Geometry check sheet. Reference: the model listing, model coordinates, mm. A direction names the side the tool comes from. Give positions to 0.01 mm unless a question says otherwise; leave off trailing zeros. Loops run counter-clockwise (first coordinate to the right, second up) from the corner with the lowest first, then second, coordinate; pieces in that order, holes last. Notation, with made-up numbers: (-22.5, -3) -> (29.5, -3) arc R24 ccw to (29.5, 8) -> close; hole circle Ø1 at (73.25, 60). An arc over 180 degrees is marked (long way). Write item = value, one per line. Start each with the question number.
```python
from build123d import *

# Parameters (mm, degrees)
SKETCH1_W           = 253.301246
SKETCH1_H           = 124.905262
BOSS_EXTRUDE1_DEPTH = 13.704316
SKETCH3_R           = 11.68527
BOSS_EXTRUDE6_DEPTH = 133.294628
SKETCH4_R           = 13.935202
BOSS_EXTRUDE7_DEPTH = 24.061166
SKETCH2_R           = 15.942437
BOSS_EXTRUDE8_DEPTH = 14.713204


with BuildPart() as part:
    # Sketch1 → Boss-Extrude1 (new body)
    with BuildSketch(Plane(origin=(0, 0, 0), x_dir=(1, 0, 0), z_dir=(0, 1, 0))):
        Rectangle(SKETCH1_W, SKETCH1_H)
    extrude(amount=BOSS_EXTRUDE1_DEPTH)

    # Sketch3 → Boss-Extrude6 (add)
    with BuildSketch(Plane.XY.offset(66.647314)):
        with Locations((131.1274492, 7.338568)):
            Circle(SKETCH3_R)
    boss_extrude6 = extrude(amount=-BOSS_EXTRUDE6_DEPTH)

    # Sketch4 → Boss-Extrude7 (add)
    with BuildSketch(Plane(origin=(47.4016832, 0, 0), x_dir=(0, 0, -1), z_dir=(1, 0, 0))):
        with BuildLine():
            Line((-44.216574, 0), (44.216574, 0))
            ThreePointArc((44.216574, 0), (0, -44.216574), (-44.216574, 0))
        make_face()
        with Locations(Location((0, -19.057366, 0), (0, 0, 180))):
            Circle(SKETCH4_R, mode=Mode.SUBTRACT)
    boss_extrude7 = extrude(amount=BOSS_EXTRUDE7_DEPTH)

    # Sketch2 → Boss-Extrude8 (add)
    with BuildSketch(Plane(origin=(127.120142, 0, 0), x_dir=(0, 0, -1), z_dir=(1, 0, 0))):
        with BuildLine():
            Line((-62.49035, 5.388102), (62.49035, 5.388102))
            Line((62.49035, 5.388102), (53.638831, 151.624284))
            ThreePointArc((53.638831, 151.624284), (44.950710882, 161.858546774), (32.082613, 165.6842))
            Line((32.082613, 165.6842), (-32.082613, 165.6842))
            ThreePointArc((-32.082613, 165.6842), (-44.950710882, 161.858546774), (-53.638831, 151.624284))
            Line((-53.638831, 151.624284), (-62.49035, 5.388102))
        make_face()
        with Locations(Location((0, 104.354376, 0), (0, 0, 180))):
            Circle(SKETCH2_R, mode=Mode.SUBTRACT)
    boss_extrude8 = extrude(amount=BOSS_EXTRUDE8_DEPTH)

    # Mirror5: Boss-Extrude6, Boss-Extrude7, Boss-Extrude8 across plane
    add(boss_extrude6.mirror(Plane(origin=(0, 0, 0), x_dir=(0, 0, 1), z_dir=(1, 0, 0))))
    add(boss_extrude7.mirror(Plane(origin=(0, 0, 0), x_dir=(0, 0, 1), z_dir=(1, 0, 0))))
    add(boss_extrude8.mirror(Plane(origin=(0, 0, 0), x_dir=(0, 0, 1), z_dir=(1, 0, 0))))


solid = part.part
```
1) Draft check along Y on faces 4 (the cylindrical face through (59.264, -5.454, -3.021)), 5 (the flat face through (-2, 7, 62.453)), 6 (the cylindrical face through (59.264, -44.206, -0.972)), 7 (the cylindrical face through (-134.374, 161.962, 44.791)). Enter one of: released by +Y, released by -Y, zero draft, split by the parting line, or undercut.
2) Thickness scan on line 1 (X direction, y = 93, z = 35.5); line 2 (Y direction, x = 66.5, z = 0); line 3 (Y direction, x = 96, z = 53). Record the ranges inside material, lowest first.
3) Depth check by flat-ended pin: pin 1 Ø8 at (x, z) = (-92.5, -40.5) entering from +Y; pin 2 Ø2 at (x, z) = (51, 7.5) entering from -Y; pin 3 Ø4 at (x, y) = (89.5, 7) entering from -Z. Enter the tip coordinate at first touch or a pass-through.
4) Section check C-C (x = 59.5). Enter the section's corners in (y, z), plus the area to 3 significant figures.
5) Section check B-B (z = 21). Enter the section's corners in (x, y).
6) Section check D-D (z = 0). Give the number of separate pieces and of enclosed holes in the cut face, plus the area to 3 significant figures.
7) Tool access check on faces 1 (the flat face through (-47.402, -7, 9)), 2 (the flat face through (-141.833, 73, 1)), 3 (the flat face through (141.833, 73, 1)). Record the directions out of +Z, -Z, +X, -X, +Y, -Y that give a thin tool (end or side, any length) a straight path to the whole face; none if there is none.
8) Section check A-A (y = 146). Enter the section's corners in (x, z), plus the area to 3 significant figures.
Check result:
q1.face_4 = undercut
q1.face_5 = zero draft
q1.face_6 = released by -Y
q1.face_7 = released by +Y
q2.line_1 = -141.83 to -127.12, 127.12 to 141.83
q2.line_2 = -44.22 to -32.99, -5.12 to 13.7
q2.line_3 = 0 to 13.7
q3.pin_1 = 13.7
q3.pin_2 = -43.74
q3.pin_3 = -62.45
q4.outline = (0, -62.45) -> (13.7, -62.45) -> (13.7, 62.45) -> (0, 62.45) -> (0, 44.22) arc R44.22 ccw to (0, -44.22) -> close; hole circle Ø27.87 at (-19.06, 0)
q4.area = 4,170 mm2
q5.outline = (-141.83, 12.02) arc R11.69 ccw to (-122.03, 0) -> (-71.46, 0) -> (-71.46, -38.91) -> (-47.4, -38.91) -> (-47.4, 0) -> (47.4, 0) -> (47.4, -38.91) -> (71.46, -38.91) -> (71.46, 0) -> (122.03, 0) arc R11.69 ccw to (141.83, 12.02) -> (141.83, 165.68) -> (127.12, 165.68) -> (127.12, 18.32) arc R11.69 ccw to (121.33, 13.7) -> (-121.33, 13.7) arc R11.69 ccw to (-127.12, 18.32) -> (-127.12, 165.68) -> (-141.83, 165.68) -> close
q6.separate_pieces = 5
q6.enclosed_holes = 0
q6.area = 8,360 mm2
q7.face_1 = +Z, -Z, -Y
q7.face_2 = +Z, -Z, -X, +Y
q7.face_3 = +Z, -Z, +X, +Y
q8.outline = (-141.83, -53.98) -> (-127.12, -53.98) -> (-127.12, 53.98) -> (-141.83, 53.98) -> close; (127.12, -53.98) -> (141.83, -53.98) -> (141.83, 53.98) -> (127.12, 53.98) -> close
q8.area = 3,180 mm2
